from build123d import *

# Parameters (mm, degrees)
RESSALTO_EXTRUS_O9_DEPTH = 6


with BuildPart() as part:
    # Esboço1 → Ressalto-extrusão9 (new body)
    with BuildSketch(Plane(origin=(0, 0, 0), x_dir=(1, 0, 0), z_dir=(0, 1, 0))):
        Polygon((-40, -6), (-40, 0), (-60, 0), (-60, -30.999999612), (-31, -30.999999612), (-31, -42.999999612), (-31, -65.999999612), (-31, -88.999999612), (-31, -100.999999612), (-60, -100.999999612), (-60, -131.999999612), (-40, -131.999999612), (-40, -125.999999612), (-30, -125.999999612), (-30, -131.999999612), (-10, -131.999999612), (-10, -125.999999612), (0, -125.999999612), (0, -131.999999612), (20, -131.999999612), (20, -95.999999612), (14, -95.999999612), (14, -75.999999612), (20, -75.999999612), (20, -55.999999612), (14, -55.999999612), (14, -36), (20, -36), (20, 0), (0, 0), (0, -6), (-10, -6), (-10, 0), (-30, 0), (-30, -6), align=None)
        Polygon((-31, -65.999999612), (-31, -42.999999612), (-54, -42.999999612), (-54, -55.999999612), (-60, -55.999999612), (-60, -65.999999612), align=None)
        Polygon((-31, -88.999999612), (-31, -65.999999612), (-60, -65.999999612), (-60, -75.999999612), (-54, -75.999999612), (-54, -88.999999612), align=None)
    extrude(amount=RESSALTO_EXTRUS_O9_DEPTH)


solid = part.part
The listing builds one solid part. Answer for the finished solid, in the listing's coordinates (mm). A direction names the side the tool comes from. Coordinates: 2 decimals unless noted, no trailing zeros. Order: outer loops, then holes, each group sorted by start corner. A loop starts at its lowest first (then second) coordinate and runs counter-clockwise, first axis right, second up. Notation, with made-up numbers: (21, 51) -> (35, 51) arc R21 cw to (35, 84) -> close; hole circle Ø3 at (61.25, -3.75). An arc over 180 degrees is marked (long way). Answer in a Markdown table with one row per item. Add a question column.
Item 1: Find the intervals of material crossed by L1, parallel to Z at x = -44, y = 0.65; L2, parallel to Z at x = -33.5, y = 4.3; L3, parallel to X at y = 2.8, z = 81, in increasing order. Write a range as from..to.
Item 2: Each of these flat-tipped pins is pushed along its axis until it touches: P1, Ø3, axis at x = -35.5, y = 3.5, coming from the -Z side; P2, Ø1.5, axis at x = -31, y = 3.5, coming from the +Z side. Where does it stop, or does it pass through?
Item 3: Find section C-C (x = -43.5). Write down the section's boundary in (y, z), then the cut area to 3 significant figures.
Item 4: Find section A-A (x = -33). Write down the section's boundary in (y, z), then the cut area to 3 significant figures.
Item 5: Which of the six approach directions +Z, -Z, +X, -X, +Y, -Y give full straight-line access (tool end or side, diameter ignored) to faces 1 (the face through (-40, 3, 3)), 2 (the face through (-40, 3, 129)), 3 (the face through (17, 3, 56)), 4 (the face through (-60, 3, 15)), 5 (the face through (-43, 3, 89))?
Item 6: Find section B-B (x = -1.5). Write down the section's boundary in (y, z).
Item 7: Determine the mould class of faces 6 (the face through (-20, 3, 132)), 7 (the face through (17, 3, 36)), 8 (the face through (-30, 3, 3)) for opening direction Z: +Z half, -Z half, draft (parallel to the pull), parting line (faces both ways), or undercut.
Result set:
| question | item | result |
|---|---|---|
| 1 | L1 | z = 0..31, 43..89, 101..132 |
| 1 | L2 | z = 6..31, 43..89, 101..126 |
| 1 | L3 | x = -54..14 |
| 2 | P1 | stops at z = 6 |
| 2 | P2 | stops at z = 126 |
| 3 | outline | (0, 0) -> (6, 0) -> (6, 31) -> (0, 31) -> close; (0, 43) -> (6, 43) -> (6, 89) -> (0, 89) -> close; (0, 101) -> (6, 101) -> (6, 132) -> (0, 132) -> close |
| 3 | area | 648 mm² |
| 4 | outline | (0, 6) -> (6, 6) -> (6, 31) -> (0, 31) -> close; (0, 43) -> (6, 43) -> (6, 89) -> (0, 89) -> close; (0, 101) -> (6, 101) -> (6, 126) -> (0, 126) -> close |
| 4 | area | 576 mm² |
| 5 | face 1 | -Z, +Y, -Y |
| 5 | face 2 | +Z, +Y, -Y |
| 5 | face 3 | +X, +Y, -Y |
| 5 | face 4 | +Z, -Z, -X, +Y, -Y |
| 5 | face 5 | -X, +Y, -Y |
| 6 | outline | (0, 6) -> (6, 6) -> (6, 126) -> (0, 126) -> close |
| 7 | face 6 | +Z half |
| 7 | face 7 | undercut |
| 7 | face 8 | draft |
